Could you check a few things on this model? Use its own coordinates, in mm. Face numbers are marked on the shaded views. Coordinates: 2 decimals unless noted, no trailing zeros. Write each loop counter-clockwise with the first axis right and the second up, starting at its lowest first coordinate (ties: lowest second). Pieces come first, ordered by that corner, then holes.
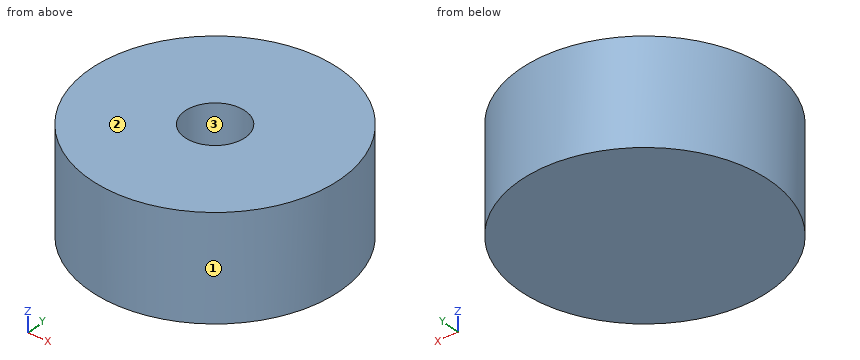
```python
from build123d import *

# Parameters (mm, degrees)
SKETCH_R    = 30
PAD_DEPTH   = 25
SKETCH001_R = 7.25
HOLE_DEPTH  = 15.643761
HOLE_TIPS_R = 7.25


with BuildPart() as part:
    # Sketch → Pad (new body)
    with BuildSketch(Plane.XY):
        Circle(SKETCH_R)
    extrude(amount=-PAD_DEPTH)

    # Sketch001 (on Face2 of Pad) → Hole (cut)
    with BuildSketch(Plane.XY):
        Circle(SKETCH001_R)
    extrude(amount=-HOLE_DEPTH, mode=Mode.SUBTRACT)

    # Hole tips → Hole tip 1 section 0
    with BuildSketch(Plane.XY.offset(-15.643761), mode=Mode.PRIVATE) as hole_tip_1_s0:
        Circle(HOLE_TIPS_R)
    loft([hole_tip_1_s0.sketch, Vertex(0, 0, -20)], mode=Mode.SUBTRACT)


solid = part.part
```
Item 1: If I drill on line 1 along Y through (x, z) = (0, -8.75); line 2 along Y through (x, z) = (0, -23.25); line 3 along X through (y, z) = (-1.5, -15.25), over which ranges is the centre line in solid material (lowest first)?
Item 2: I want a section at D-D, the plane z = -18.5. List the corners of the cut face in (x, y) for me.
Item 3: I want a section at C-C, the plane x = -9. List the corners of the cut face in (y, z) for me, then the cut area to 3 significant figures.
Item 4: If we mould it in two halves opening along X, with no side actions, what happens to the marked faces 1, 2 and 3? For each: released by +X, released by -X, zero draft, split by the parting line, or undercut.
Item 5: I want a section at B-B, the plane y = -17. List the corners of the cut face in (x, z) for me.
Item 6: I want a section at A-A, the plane z = -9. List the corners of the cut face in (x, y) for me, then the cut area to 3 significant figures.
Item 7: Will these pins go through, and if not, where does the flat tip stop? pin 1 Ø6 at (y, z) = (-18.5, -7) entering from +X; pin 2 Ø6 at (y, z) = (-23, -6.5) entering from -X; pin 3 Ø6 at (x, z) = (-22, -6.5) entering from +Y.
Taken from the geometry:
1. line 1: y = -30 to -7.25, 7.25 to 30
1. line 2: y = -30 to 30
1. line 3: x = -29.96 to -7.09, 7.09 to 29.96
2. outline: circle Ø60 at (0, 0); hole circle Ø4.99 at (0, 0)
3. outline: (-28.62, -25) - (28.62, -25) - (28.62, 0) - (-28.62, 0) - close
3. area: 1,430 mm2
4. face 1: split by the parting line
4. face 2: zero draft
4. face 3: undercut
5. outline: (-24.72, -25) - (24.72, -25) - (24.72, 0) - (-24.72, 0) - close
6. outline: circle Ø60 at (0, 0); hole circle Ø14.5 at (0, 0)
6. area: 2,660 mm2
7. pin 1: stops at x = 25.69
7. pin 2: stops at x = -22.36
7. pin 3: stops at y = 23.22
